Input: part model. Units: mm. Frame: model coordinates. Face numbers are marked on the shaded views. A direction names the side the tool comes from. Coordinates: 2 decimals unless noted, no trailing zeros. Order: outer loops, then holes, each group sorted by start corner. A loop starts at its lowest first (then second) coordinate and runs counter-clockwise, first axis right, second up. Notation, with made-up numbers: (17, -21.5) -> (66, -21.5) arc R33 ccw to (66, 14.5) -> close; hole circle Ø8 at (59.25, 22). An arc over 180 degrees is marked (long way). One line per item, written item: value. Start each with the question number.
from build123d import *

# Parameters (mm, degrees)
EXTRUDE_1_DEPTH = 5
SKETCH_3_R      = 2.640227158
SKETCH_3_R_2    = 3.578323713
EXTRUDE_2_DEPTH = 3
FILLET_3_R      = 2


with BuildPart() as part:
    # 草圖1 → 填料-伸長1 (new body)
    with BuildSketch(Plane.XY):
        with BuildLine():
            Line((0, 0), (-12.2, 0))
            Line((-12.2, 0), (-12.2, -22.5))
            Line((-12.2, -22.5), (0, -22.5))
            Line((0, -22.5), (0, -62.5))
            ThreePointArc((0, -62.5), (-1.561204321, -64.451270958), (-3.807458352, -63.356209266))
            Line((-3.807458352, -63.356209266), (-15.358968834, -38.970962655))
            ThreePointArc((-15.358968834, -38.970962655), (-16.797094897, -34.796826792), (-17.284385317, -30.408869998))
            Line((-17.284385317, -30.408869998), (-17.284385317, 5))
            ThreePointArc((-17.284385317, 5), (-8.642192658, 13.642192658), (0, 5))
            Line((0, 5), (0, 0))
        make_face()
    extrude(amount=EXTRUDE_1_DEPTH)

    # 草圖3 → 填料-伸長2 (add)
    with BuildSketch(Plane.XY.offset(5)):
        with Locations(Location((-7.938901353, -32.425782639, 0), (0, 0, 180))):
            Circle(SKETCH_3_R)
        with Locations(Location((-6.788376637, -42.772023111, 0), (0, 0, 180))):
            Circle(SKETCH_3_R_2)
    extrude(amount=EXTRUDE_2_DEPTH)

    # 圓角3
    fillet_3_edges = [part.edges().sort_by_distance(p)[0] for p in [
        (-6.1, -22.5, 0),
        (0, -42.5, 0),
        (-1.561204321, -64.451270958, 0),
        (-9.583213593, -51.163585961, 0),
        (-16.797094897, -34.796826792, 0),
        (-17.284385317, -12.704434999, 0),
        (-8.642192658, 13.642192658, 0),
        (0, 2.5, 0),
        (-6.1, 0, 0),
        (-12.2, -11.25, 0),
    ]]
    fillet(fillet_3_edges, radius=FILLET_3_R)


solid = part.part
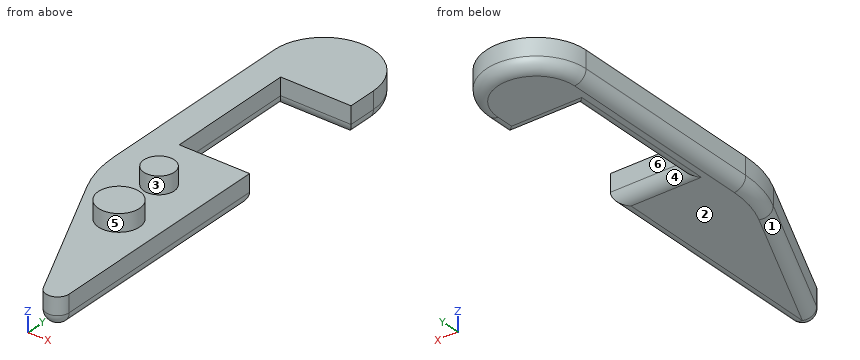
1) Section query B-B, the plane y = -18. Return the cut outline in (x, z).
2) Pin query (flat end, axial travel): pin 1 Ø0.9 at (y, z) = (-11, 4) entering from +X; pin 2 Ø3.5 at (x, z) = (-5, 3) entering from +Y; pin 3 Ø1 at (x, z) = (-12.5, 5) entering from -Y. Return the tip coordinate at first contact, or that it passes through.
3) Section query C-C, the plane z = 7.25. Return the cut outline in (x, y).
4) Mould query, pull axis Y, two halves, no side actions, for the marked faces 1, 2 and 3. Classes: +Y half, -Y half, draft (parallel to the pull), parting line (faces both ways), or undercut.
5) Ray query, line 1 along Z through (x, y) = (-15, -22); line 2 along Y through (x, z) = (-2.5, 2); line 3 along Y through (x, z) = (-3.5, 1.5). Return the intervals inside material, ascending. Write a range as from..to.
6) Access query for the marked faces 4, 5 and 6. Directions: +Z, -Z, +X, -X, +Y, -Y. A direction counts if a zero-diameter tool reaches every point of the face in a straight line with its end or side. Return the directions, or none.
7) Section query A-A, the plane z = 3.25. Return the cut outline in (x, y), plus the area to 3 significant figures.
Entries:
1. outline: (-17.28, 2) arc R2 ccw to (-15.28, 0) -> (-14.2, 0) arc R2 ccw to (-12.2, 2) -> (-12.2, 5) -> (-17.28, 5) -> close
2. pin 1: stops at x = -12.2
2. pin 2: stops at y = 13.43
2. pin 3: stops at y = -46.06
3. outline: circle Ø5.28 at (-7.94, -32.43); circle Ø7.16 at (-6.79, -42.77)
4. face 1: -Y half
4. face 2: draft
4. face 3: undercut
5. line 1: z = 0..5
5. line 2: y = -64.44..-22.5, 0..11.08
5. line 3: y = -63.72..-22.56, 0.06..11.87
6. face 4: -Z, +X
6. face 5: +Z
6. face 6: +Z, -Z, +X
7. outline: (-17.28, -30.41) arc R20 ccw to (-15.36, -38.97) -> (-3.81, -63.36) arc R2 ccw to (0, -62.5) -> (0, -22.5) -> (-12.2, -22.5) -> (-12.2, 0) -> (0, 0) -> (0, 5) arc R8.64 ccw to (-17.28, 5) -> close
7. area: 834 mm2
